Part model, mm, in its own coordinate system. Coordinates: 2 decimals unless noted, no trailing zeros. Loops run counter-clockwise (first coordinate to the right, second up) from the corner with the lowest first, then second, coordinate; pieces in that order, holes last. Notation, with made-up numbers: (58.5, -29.5) - (76.5, -29.5) arc R25 cw to (76.5, -12.5) - close; hole circle Ø6 at (-23.75, 31). An arc over 180 degrees is marked (long way). Use a Markdown table: item, result. Add a question column.
1) Drop a flat-ended pin along its axis: P1, Ø6, axis at x = 12, z = 5, coming from the -Y side. Give the stop position or say it passes through.
2) Band-saw the part on A-A (x = 3). Give the cut face in (y, z).
3) Probe probe 1 along Z at (x, y) = (5.5, 1.15); probe 2 along X at (y, z) = (0.2, 20); probe 3 along X at (y, z) = (0.2, 16). List the from-to ranges inside material, lowest first. Write a range as [from, to].
4) Band-saw the part on C-C (y = 0.5). Give the cut face in (x, z).
5) Band-saw the part on B-B (z = 3). Give the cut face in (x, y).
Autodesk Fusion 360 part; units mm, degrees
sketch "Sketch9" plane through (0, 0, 0) normal (0, 1, 0) x (1, 0, 0)
  line L0 (-6, 8.1973) -> (26, 8.1973)
  line L1 (26, 8.1973) -> (26, -26.8027)
  line L2 (26, -26.8027) -> (-6, -26.8027)
  line L3 (-6, -26.8027) -> (-6, 8.1973)
  line L4 (10, 8.1973) -> (10, -16.3027)
  line L5 (22.4349, 8.1973) -> (22.4349, -19.3027)
  line L6 (-2.5651, 8.1973) -> (-2.5651, -19.3027)
  circle A0 centre (-2.5651, -19.3027) radius 1.5
  circle A1 centre (22.4349, -19.3027) radius 1.5
  line L7 (-2.5651, -19.3027) -> (22.4349, -19.3027)
  line L8 (10, -16.3027) -> (9.4349, -16.3027)
  line L9 (-2.5651, -16.3027) -> (22.4349, -16.3027)
  line L10 (9.9349, 0.6973) -> (-1.5651, 0.6973)
  line L11 (9.9349, 0.6973) -> (21.4349, 0.6973)
  line L12 (-1.5651, 0.6973) -> (-1.5651, -16.3027)
  line L13 (21.4349, 0.6973) -> (21.4349, -16.3027)
  dimension "d91" = 35
  dimension "d92" = 32
  dimension "d124" = 24.5
  dimension "d125" = 27.5
  dimension "d129" = 27.5
  dimension "d130" = 3
  dimension "d131" = 3
  dimension "d132" = 25
  dimension "d134" = 11.5
  dimension "d135" = 11.5
extrude "Extrude14" add sketch "Sketch9" along normal blind 1.5 contours L0 L1 L2 L3 L5 L6 A0 A1 L7 | L0 L4 L6 L9 L10 L11 L12 | L0 L4 L5 L9 L11 L13 | L5 L6 A0 A1 L7 L8 L9
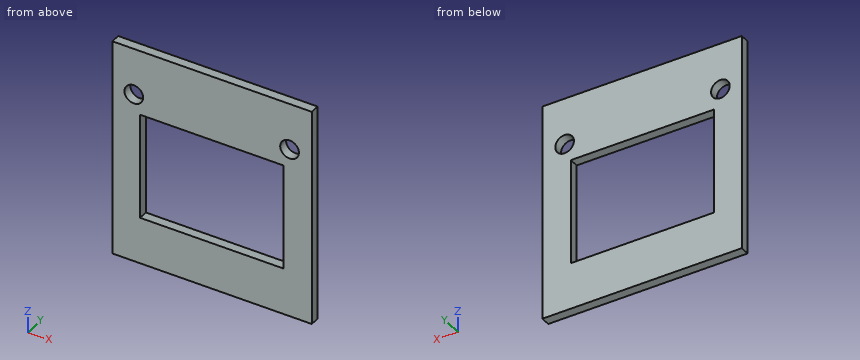
Answer block:
| question | item | result |
|---|---|---|
| 1 | P1 | through |
| 2 | outline | (0, -8.2) - (1.5, -8.2) - (1.5, -0.7) - (0, -0.7) - close; (0, 16.3) - (1.5, 16.3) - (1.5, 26.8) - (0, 26.8) - close |
| 3 | probe 1 | [-8.2, -0.7], [16.3, 26.8] |
| 3 | probe 2 | [-6, -3.89], [-1.24, 21.11], [23.76, 26] |
| 3 | probe 3 | [-6, -1.57], [21.43, 26] |
| 4 | outline | (-6, -8.2) - (26, -8.2) - (26, 26.8) - (-6, 26.8) - close; hole circle Ø3 at (-2.57, 19.3); hole (-1.57, -0.7) - (21.43, -0.7) - (21.43, 16.3) - (-1.57, 16.3) - close; hole circle Ø3 at (22.43, 19.3) |
| 5 | outline | (-6, 0) - (-1.57, 0) - (-1.57, 1.5) - (-6, 1.5) - close; (21.43, 0) - (26, 0) - (26, 1.5) - (21.43, 1.5) - close |
